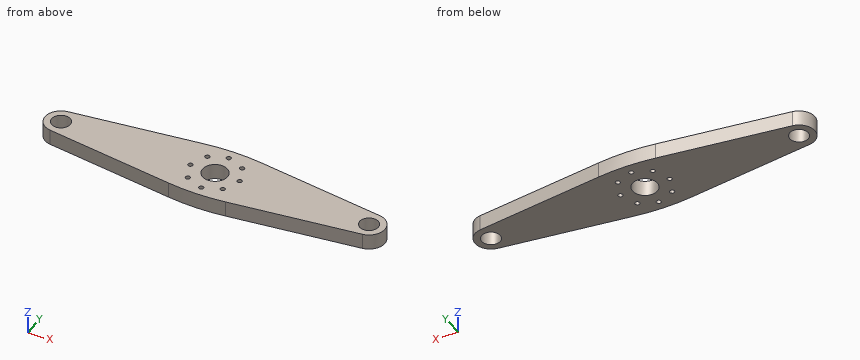
```python
from build123d import *

# Parameters (mm, degrees)
SZKIC1_R                    = 4
SZKIC1_R_2                  = 0.75
SZKIC1_R_3                  = 3
DODANIE_WYCI_GNI_CIE1_DEPTH = 5


with BuildPart() as part:
    # Szkic1 → Dodanie-wyciągnięcie1 (new body)
    with BuildSketch(Plane.XY):
        with BuildLine():
            Line((-50.67287635, 5.055665151), (-9.235111676, 10.570763761))
            ThreePointArc((-9.235111676, 10.570763761), (0, 11.182632843), (9.235111676, 10.570763761))
            Line((9.235111676, 10.570763761), (50.67287635, 5.055665151))
            ThreePointArc((50.67287635, 5.055665151), (55.100246338, 0), (50.67287635, -5.055665151))
            Line((50.67287635, -5.055665151), (9.235111676, -10.570763761))
            ThreePointArc((9.235111676, -10.570763761), (0, -11.182632843), (-9.235111676, -10.570763761))
            Line((-9.235111676, -10.570763761), (-50.67287635, -5.055665151))
            ThreePointArc((-50.67287635, -5.055665151), (-55.100246338, 0), (-50.67287635, 5.055665151))
        make_face()
        Circle(SZKIC1_R, mode=Mode.SUBTRACT)
        with Locations((-5.656854249, 5.656854249)):
            Circle(SZKIC1_R_2, mode=Mode.SUBTRACT)
        with Locations((-8, 0)):
            Circle(SZKIC1_R_2, mode=Mode.SUBTRACT)
        with Locations((0, 8)):
            Circle(SZKIC1_R_2, mode=Mode.SUBTRACT)
        with Locations((5.656854249, 5.656854249)):
            Circle(SZKIC1_R_2, mode=Mode.SUBTRACT)
        with Locations((-50, 0)):
            Circle(SZKIC1_R_3, mode=Mode.SUBTRACT)
        with Locations((50, 0)):
            Circle(SZKIC1_R_3, mode=Mode.SUBTRACT)
        with Locations((8, 0)):
            Circle(SZKIC1_R_2, mode=Mode.SUBTRACT)
        with Locations((5.656854249, -5.656854249)):
            Circle(SZKIC1_R_2, mode=Mode.SUBTRACT)
        with Locations((0, -8)):
            Circle(SZKIC1_R_2, mode=Mode.SUBTRACT)
        with Locations((-5.656854249, -5.656854249)):
            Circle(SZKIC1_R_2, mode=Mode.SUBTRACT)
    extrude(amount=DODANIE_WYCI_GNI_CIE1_DEPTH)


solid = part.part
```
Design review of the part built by this model. Coordinates are the model's own, in mm. Coordinates: 2 decimals unless noted, no trailing zeros. Answer as a JSON object with one key per item and string values.
Item 1: Wall thickness on probe 1 along Y at (x, z) = (0, 3.4); probe 2 along X at (y, z) = (1, 2.55); probe 3 along Y at (x, z) = (-5, 3.3): over which ranges is each line inside the solid? List them lowest first.
Outcome:
{"probe 1": "-11.18 to -8.75, -7.25 to -4, 4 to 7.25, 8.75 to 11.18", "probe 2": "-55 to -52.83, -47.17 to -3.87, 3.87 to 47.17, 52.83 to 55", "probe 3": "-11 to -6.02, -5.29 to 5.29, 6.02 to 11"}
Item 2: Insertion check: pin 1 Ø0.9 at (x, y) = (-8, 0) entering from +Z; pin 2 Ø3 at (x, z) = (-27.5, 3.5) entering from -Y; pin 3 Ø1 at (x, z) = (-9.5, 1.5) entering from -Y; pin 4 Ø1 at (x, z) = (-4, 3.5) entering from -Y. Each pin has a flat end and moves straight along its axis. Give the tip position at first contact, or say it passes through.
Outcome:
{"pin 1": "through", "pin 2": "y = -8.34", "pin 3": "y = -10.6", "pin 4": "y = -11.1"}
Item 3: Add section A-A, the plane z = 2.15. State how many separate pieces and enclosed holes the cut face has, and give its area (3 significant figures).
Outcome:
{"separate pieces": "1", "enclosed holes": "11", "area": "1,650 mm²"}
